The model under review builds one solid part; all positions refer to its coordinate system, in mm. Give positions to 0.01 mm unless a question says otherwise; leave off trailing zeros. Order: outer loops, then holes, each group sorted by start corner. A loop starts at its lowest first (then second) coordinate and runs counter-clockwise, first axis right, second up. Notation, with made-up numbers: (68, -29.5) - (79, -29.5) arc R20 cw to (79, -25.5) - close; hole circle Ø10 at (-33.5, -18.75). An arc over 180 degrees is marked (long way). Use CSV: the item, a comma, the result in double quotes.
```python
from build123d import *

# Parameters (mm, degrees)
SKETCH1_W           = 276
SKETCH1_H           = 400
BOSS_EXTRUDE1_DEPTH = 3
SKETCH2_W           = 28
SKETCH2_H           = 192
CUT_EXTRUDE1_DEPTH  = 25


with BuildPart() as part:
    # Sketch1 → Boss-Extrude1 (new body)
    with BuildSketch(Plane(origin=(0, 0, 0), x_dir=(0, 0, -1), z_dir=(1, 0, 0))):
        with Locations((-123.692307692, -9.461538462)):
            Rectangle(SKETCH1_W, SKETCH1_H)
    extrude(amount=BOSS_EXTRUDE1_DEPTH)

    # Sketch2 → Cut-Extrude1 (cut)
    with BuildSketch(Plane(origin=(0, 0, 0), x_dir=(0, 0, -1), z_dir=(1, 0, 0))):
        with Locations((0.307692308, -9.461538462)):
            Rectangle(SKETCH2_W, SKETCH2_H)
        with Locations((-247.692307692, -9.461538462)):
            Rectangle(SKETCH2_W, SKETCH2_H)
    extrude(amount=CUT_EXTRUDE1_DEPTH, mode=Mode.SUBTRACT)


solid = part.part
```
Item 1: Clearance check with flat-ended pins moving along their axes: pin 1 (8 mm diameter, centred on y = 136, z = 49, fed in from -X); pin 2 (0.9 mm diameter, centred on x = 2, y = -10.5, fed in from -Z); pin 3 (1.5 mm diameter, centred on x = 2, y = 61.5, fed in from +Z). State where each tip first meets the part, or that it passes through.
Results list:
pin 1,"stops at x = 0"
pin 2,"stops at z = 13.69"
pin 3,"stops at z = 233.69"
Item 2: Wall thickness on L1, parallel to Z at x = 2.7, y = 11; L2, parallel to Y at x = 2.1, z = 3: over which ranges is each line inside the solid? List them lowest first.
Results list:
L1,"z = 13.69 to 233.69"
L2,"y = -209.46 to -105.46, 86.54 to 190.54"
Item 3: Take a section at C-C, the plane y = 41. Give the boundary of the cut face in (x, z).
Results list:
outline,"(0, 13.69) - (3, 13.69) - (3, 233.69) - (0, 233.69) - close"
Item 4: Take a section at B-B, the plane x = 2.3. Give the boundary of the cut face in (y, z), and give its area (3 significant figures).
Results list:
outline,"(-209.46, -14.31) - (-105.46, -14.31) - (-105.46, 13.69) - (86.54, 13.69) - (86.54, -14.31) - (190.54, -14.31) - (190.54, 261.69) - (86.54, 261.69) - (86.54, 233.69) - (-105.46, 233.69) - (-105.46, 261.69) - (-209.46, 261.69) - close"
area,"99,600 mm2"
Item 5: Take a section at A-A, the plane z = 242. Give the boundary of the cut face in (x, y).
Results list:
outline,"(0, -209.46) - (3, -209.46) - (3, -105.46) - (0, -105.46) - close; (0, 86.54) - (3, 86.54) - (3, 190.54) - (0, 190.54) - close"
